Can you work these out from the drawing? Everything is in mm from the part's minimum corner. A direction names the side the tool comes from. Coordinates: 2 decimals unless noted, no trailing zeros. Write each loop counter-clockwise with the first axis right and the second up, starting at its lowest first coordinate (ties: lowest second). Pieces come first, ordered by that corner, then holes.
(1) Thinking about a two-plate mould opening in Z: for the marked faces 3, 4 and 5, which applies, released by +Z, released by -Z, zero draft, split by the parting line, or undercut?
(2) Imagine slicing it at D-D, the plane x = 13. List the corners of the cut face in (y, z) for me, plus the area to 3 significant figures.
(3) Imagine slicing it at C-C, the plane y = 21.75. List the corners of the cut face in (x, z) for me.
(4) For pin 1 Ø0.5 at (x, z) = (10, 3.5) entering from -Y, with a flat end and sliding along its axis, tell me the tip position at first contact or that it passes through.
(5) Which directions (+Z, -Z, +X, -X, +Y, -Y) give clear straight access to the entire face, cutting with the end or side of a thin tool? Please do the marked faces 1 and 2.
(6) Imagine slicing it at A-A, the plane y = 4. List the corners of the cut face in (x, z) for me (1 decimal).
(7) Imagine slicing it at B-B, the plane z = 6.5. List the corners of the cut face in (x, y) for me.
(8) Please list where these lines run through material, in increasing order: probe 1 along Y at (x, z) = (8, 3.75); probe 2 along Z at (x, y) = (7, 13.5) (1 decimal); probe 3 along Z at (x, y) = (9.25, 6.5).
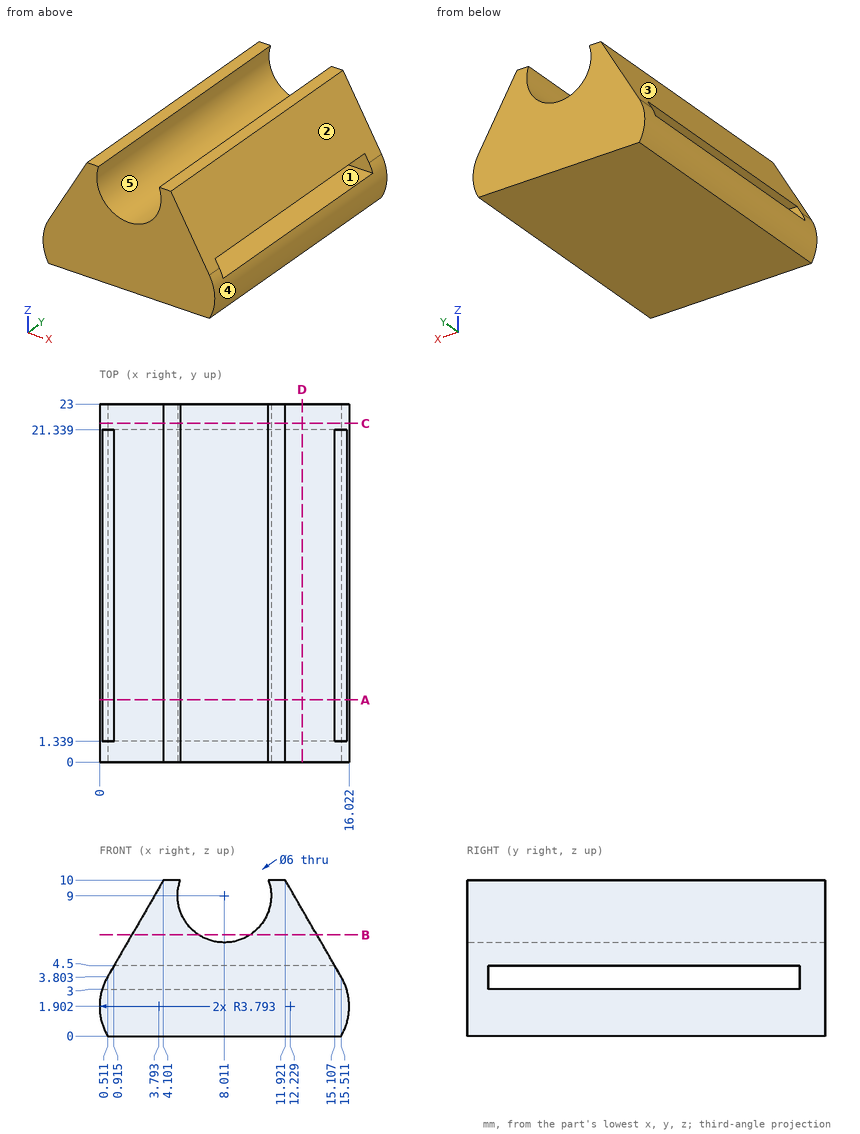
Recorded:
1. face 3: released by +Z
1. face 4: split by the parting line
1. face 5: undercut
2. outline: (0, 0) - (23, 0) - (23, 8.14) - (0, 8.14) - close; hole (1.34, 3) - (21.34, 3) - (21.34, 4.5) - (1.34, 4.5) - close
2. area: 157 mm2
3. outline: (0.51, 0) - (15.51, 0) arc R3.79 ccw to (15.51, 3.8) - (11.92, 10) - (10.84, 10) arc R3 cw (long way) to (5.18, 10) - (4.1, 10) - (0.51, 3.8) arc R3.79 ccw to start
4. pin 1: stops at y = 0
5. face 1: +X, -X
5. face 2: +Z, +X, +Y, -Y
6. outline: (0.2, 3) arc R3.8 ccw to (0.5, 0) - (15.5, 0) arc R3.8 ccw to (15.9, 3) - close; (0.9, 4.5) - (15.1, 4.5) - (11.9, 10) - (10.8, 10) arc R3 cw (long way) to (5.2, 10) - (4.1, 10) - close
7. outline: (2.07, 0) - (6.35, 0) - (6.35, 23) - (2.07, 23) - close; (9.67, 0) - (13.95, 0) - (13.95, 23) - (9.67, 23) - close
8. probe 1: y = 0 to 1.34, 21.34 to 23
8. probe 2: z = 0 to 3, 4.5 to 6.2
8. probe 3: z = 0 to 3, 4.5 to 6.27
